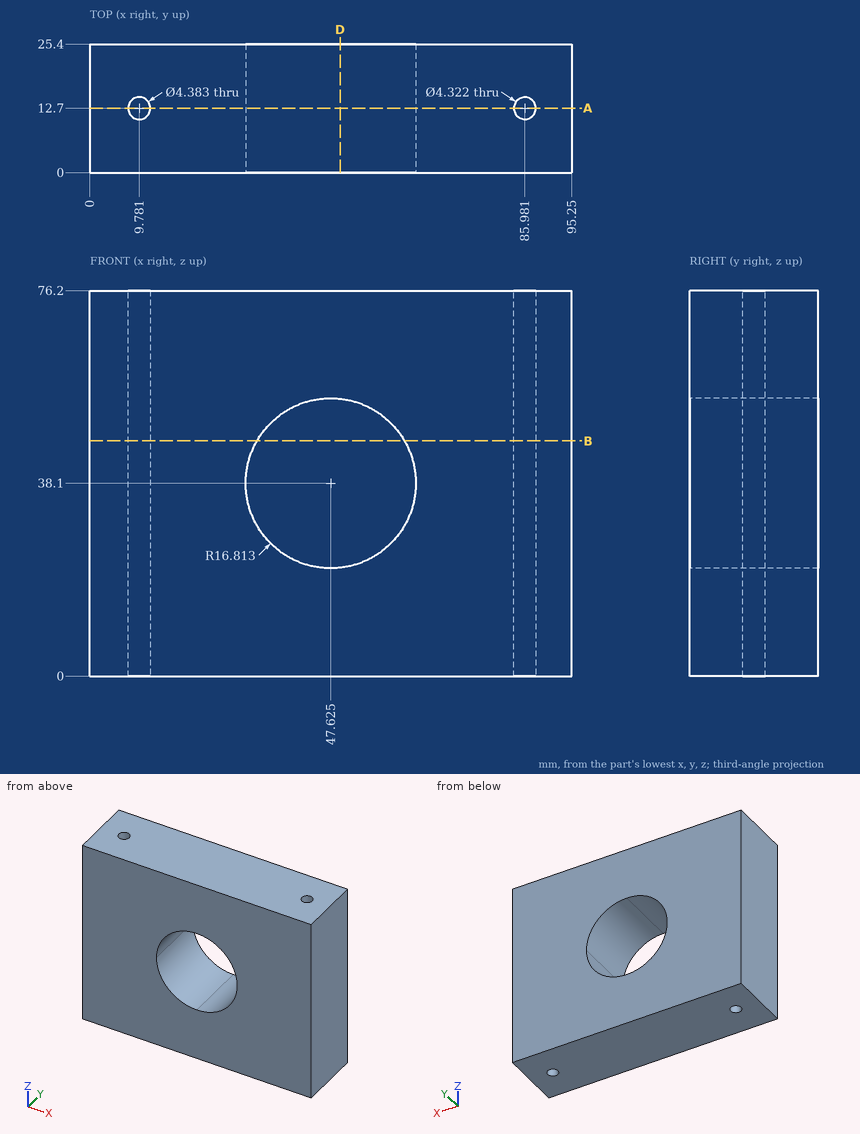
Geometry: see drawing. Coordinates: mm, zero at the bounding-box minimum. Coordinates: 2 decimals unless noted, no trailing zeros. Loops run counter-clockwise (first coordinate to the right, second up) from the corner with the lowest first, then second, coordinate; pieces in that order, holes last. Notation, with made-up numbers: (-40, 27.25) - (5, 27.25) arc R34 cw to (5, 66.25) - close; hole circle Ø6 at (88.5, -17.5). An arc over 180 degrees is marked (long way). Answer as CSV lines item,"result".
1. Section A-A (y = 12.7). Count the separate pieces of the cut face and the enclosed holes in it, then the cut area to 3 significant figures.
Established:
separate pieces,"3"
enclosed holes,"1"
area,"5,710 mm2"
2. Contact query for a flat-ended pin moving along its axis: pin 1 (3 mm diameter, centred on x = 83, z = 46, fed in from -Y). Output: stop coordinate, or through.
Established:
pin 1,"stops at y = 0"
3. Ray query, line 1 (X direction, y = 12.75, z = 58); line 2 (X direction, y = 17.75, z = 43); line 3 (Z direction, x = 62, y = 11). Return the intervals inside material, ascending.
Established:
line 1,"x = 0 to 7.59, 11.97 to 83.82, 88.14 to 95.25"
line 2,"x = 0 to 31.54, 63.71 to 95.25"
line 3,"z = 0 to 29.38, 46.82 to 76.2"
4. Section D-D (x = 49.5). Return loops of the section in (y, z).
Established:
outline,"(0, 0) - (25.4, 0) - (25.4, 21.39) - (0, 21.39) - close; (0, 54.81) - (25.4, 54.81) - (25.4, 76.2) - (0, 76.2) - close"
5. Section B-B (z = 46.5). Return loops of the section in (x, y), then the cut area to 3 significant figures.
Established:
outline,"(0, 0) - (33.06, 0) - (33.06, 25.4) - (0, 25.4) - close; (62.19, 0) - (95.25, 0) - (95.25, 25.4) - (62.19, 25.4) - close; hole circle Ø4.38 at (9.78, 12.7); hole circle Ø4.32 at (85.98, 12.7)"
area,"1,650 mm2"
